Part model, mm, in its own coordinate system. Face numbers are marked on the shaded views. Round coordinates to 2 decimals unless told otherwise and drop trailing zeros. Write each loop counter-clockwise with the first axis right and the second up, starting at its lowest first coordinate (ties: lowest second). Pieces come first, ordered by that corner, then holes.
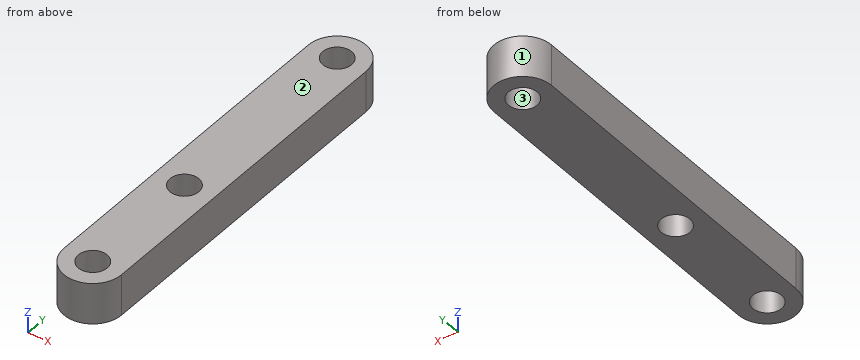
Autodesk Inventor part; units mm, degrees
ref_plane "YZ Plane" through (0, 0, 0) normal (1, 0, 0) x (0, 1, 0)
ref_plane "XZ Plane" through (0, 0, 0) normal (0, 1, 0) x (-1, 0, 0)
ref_plane "XY Plane" through (0, 0, 0) normal (0, 0, 1) x (1, 0, 0)
sketch "Sketch1" plane through (0, 0, 0) normal (0, 0, 1) x (1, 0, 0)
  circle A0 centre (0, 0) radius 3.5
  line L0 (0, 0) -> (0, 40)
  circle A1 centre (0, 40) radius 3.5
  line L1 (3.5, 40) -> (3.5, 0)
  line L2 (-3.5, 40) -> (-3.5, 0)
  dimension "d0" = 7
  dimension "d1" = 40
  dimension "d2" = 7
extrude "Extrusion1" add sketch "Sketch1" along normal blind 5
sketch "Sketch2" plane through (0, 0, 5) normal (0, 0, 1) x (1, 0, 0)
  circle A0 centre (0, 0) radius 1.75
  arc A1 (3.5, 40) -> (-3.5, 40) centre (0, 40) ccw
  circle A2 centre (0, 40) radius 1.75
  dimension "d5" = 3.5
  dimension "d6" = 3.5
extrude "Extrusion2" cut sketch "Sketch2" against normal blind 5
sketch "Sketch3" plane through (0, 0, 5) normal (0, 0, 1) x (1, 0, 0)
  line L0 (0, 0) -> (0, 15)
  circle A0 centre (0, 15) radius 1.75
  dimension "d9" = 15
  dimension "d10" = 3.5
extrude "Extrusion3" cut sketch "Sketch3" against normal blind 10
properties part number "bar"
Q1. Saw through at B-B, the plane y = 15. Write the cut outline in (x, z).
Q2. Drop flat-ended pins along their axis: P1, Ø1, axis at x = -2.5, z = 0.5, coming from the -Y side; P2, Ø2, axis at x = 0, y = 0, coming from the -Z side. Give the stop position or say it passes through.
Q3. Saw through at C-C, the plane z = 2.7. Write the cut outline in (x, y).
Q4. Two-plate mould, pull along X, no slides. Class the marked faces 1, 2 and 3: released by +X, released by -X, zero draft, split by the parting line, or undercut.
Q5. Wall check: line 1 (Y direction, x = 0, z = 2.55); line 2 (X direction, y = 15, z = 1.75); line 3 (Y direction, x = 1.25, z = 1.25). Give the ranges that are in metal, low to high.
Q6. Saw through at A-A, the plane x = 0. Write the cut outline in (y, z).
Computed:
1. outline: (-3.5, 0) - (-1.75, 0) - (-1.75, 5) - (-3.5, 5) - close; (1.75, 0) - (3.5, 0) - (3.5, 5) - (1.75, 5) - close
2. P1: stops at y = -2.87
2. P2: passes through
3. outline: (-3.5, 0) arc R3.5 ccw to (3.5, 0) - (3.5, 40) arc R3.5 ccw to (-3.5, 40) - close; hole circle Ø3.5 at (0, 0); hole circle Ø3.5 at (0, 15); hole circle Ø3.5 at (0, 40)
4. face 1: split by the parting line
4. face 2: zero draft
4. face 3: undercut
5. line 1: y = -3.5 to -1.75, 1.75 to 13.25, 16.75 to 38.25, 41.75 to 43.5
5. line 2: x = -3.5 to -1.75, 1.75 to 3.5
5. line 3: y = -3.27 to -1.22, 1.22 to 13.78, 16.22 to 38.78, 41.22 to 43.27
6. outline: (-3.5, 0) - (-1.75, 0) - (-1.75, 5) - (-3.5, 5) - close; (1.75, 0) - (13.25, 0) - (13.25, 5) - (1.75, 5) - close; (16.75, 0) - (38.25, 0) - (38.25, 5) - (16.75, 5) - close; (41.75, 0) - (43.5, 0) - (43.5, 5) - (41.75, 5) - close
